Autodesk Inventor part; units mm, degrees
ref_plane "YZ Plane" through (0, 0, 0) normal (1, 0, 0) x (0, 1, 0)
ref_plane "XZ Plane" through (0, 0, 0) normal (0, 1, 0) x (-1, 0, 0)
ref_plane "XY Plane" through (0, 0, 0) normal (0, 0, 1) x (1, 0, 0)
sketch "Sketch1" plane through (0, 0, 0) normal (0, 1, 0) x (-1, 0, 0)
  line L0 (0, 0) -> (8, 0)
  line L1 (8, -30) -> (0, -30)
  line L2 (0, -30) -> (0, 0)
  line L3 (6.25, -3.4) -> (1.75, -3.4)
  line L4 (1.75, -3.4) -> (1.75, -6.4)
  line L5 (1.75, -6.4) -> (6.25, -6.4)
  line L6 (6.25, -6.4) -> (6.25, -3.4)
  line L7 (6.25, -23.6) -> (1.75, -23.6)
  line L8 (1.75, -23.6) -> (1.75, -26.6)
  line L9 (1.75, -26.6) -> (6.25, -26.6)
  line L10 (6.25, -26.6) -> (6.25, -23.6)
  line L11 (8, 0) -> (30, -7.5)
  line L12 (30, -7.5) -> (30, -22.5)
  line L13 (30, -22.5) -> (8, -30)
  dimension "d0" = 30
  dimension "d1" = 8
  dimension "d2" = 4.5
  dimension "d3" = 3
  dimension "d4" = 3
  dimension "d5" = 17.2
  dimension "d6" = 3.4
  dimension "d7" = 1.75
  dimension "d8" = 15
  dimension "d10" = 7.5
  dimension "d11" = 22
  dimension "d12" = 22
extrude "Extrusion1" add sketch "Sketch1" along normal blind 3
sketch "Sketch2" plane through (0, 3, 0) normal (0, 1, 0) x (1, 0, 0)
  circle A0 centre (-7, 15) radius 1.3
  line L0 (-30, 22.5) -> (-30, 7.5)
  line L1 (-30, 7.5) -> (0, 7.5)
  line L2 (-30, 22.5) -> (0, 22.5)
  line L3 (-30, 7.5) -> (-14.7467, 2.3)
  line L4 (-30, 7.5) -> (-8, 0)
  line L5 (0, 0) -> (0, 30)
  line L6 (0, 2.3) -> (0, 7.5)
  line L7 (0, 2.3) -> (-14.7467, 2.3)
  line L8 (-8, 30) -> (-30, 22.5)
  line L9 (-30, 22.5) -> (-14.7467, 27.7)
  line L10 (-14.7467, 27.7) -> (0, 27.7)
  line L11 (0, 27.7) -> (0, 22.5)
  line L12 (-8, 0) -> (0, 0)
  line L13 (-1.75, 3.4) -> (-6.25, 3.4)
  line L14 (-6.25, 26.6) -> (-1.75, 26.6)
  point P0 (0, 27.7)
  dimension "d17" = 2.6
  dimension "d21" = 1.1
  dimension "d22" = 1.1
  dimension "d23" = 15
  dimension "d24" = 7
extrude "Extrusion2" add sketch "Sketch2" along normal blind 7 contours A0 | L8 L10 L5 L2 | L1 L5 L7 L3
sketch "Sketch3" plane through (0, 0, 0) normal (0, -1, 0) x (1, 0, 0)
  line L0 (-1.75, -6.4) -> (-1.75, -3.4)
  line L1 (-1.75, -3.4) -> (-6.25, -3.4)
  line L2 (-6.25, -3.4) -> (-6.25, -6.4)
  line L3 (-6.25, -6.4) -> (-1.75, -6.4)
  line L4 (-1.75, -6.4) -> (-1.75, -3.4)
  line L5 (-1.75, -26.6) -> (-1.75, -23.6)
  line L6 (-6.25, -26.6) -> (-1.75, -26.6)
  line L7 (-1.75, -23.6) -> (-6.25, -23.6)
  line L8 (-6.25, -23.6) -> (-6.25, -26.6)
  line L9 (-6.25, -26.6) -> (-1.75, -26.6)
  line L10 (-1.75, -26.6) -> (-1.75, -23.6)
  point P0 (0, 0)
extrude "Extrusion3" cut sketch "Sketch3" against normal through all
sketch "Sketch4" plane through (0, 3, 0) normal (0, 1, 0) x (1, 0, 0)
  line L0 (0, 7.5) -> (0, 22.5)
  line L1 (0, 11) -> (-4, 11)
  line L2 (-4, 11) -> (-4, 19)
  line L3 (-4, 19) -> (0, 19)
  line L4 (0, 19) -> (0, 11)
  circle A0 centre (-7, 15) radius 1.3
  line L5 (0, 7.5) -> (-30, 7.5)
  point P0 (0, 0)
  point P1 (0, 19)
  dimension "d29" = 3
  dimension "d30" = 8
  dimension "d31" = 3.5
extrude "Extrusion4" cut sketch "Sketch4" against normal through all contours L1 L2 L3 L0
fillet "Fillet1" radius 1 1 edges at (-8.3, 3, -15)
properties part number "IRMount"
Could you check a few things on this model? Use its own coordinates, in mm. A direction names the side the tool comes from. Give positions to 0.01 mm unless a question says otherwise; leave off trailing zeros. Loops run counter-clockwise (first coordinate to the right, second up) from the corner with the lowest first, then second, coordinate; pieces in that order, holes last. Notation, with made-up numbers: (36.25, 2.5) - (92.25, 2.5) arc R18 ccw to (92.25, 19.5) - close; hole circle Ø7 at (80, -13). An arc over 180 degrees is marked (long way). Answer in a Markdown table with one row per item. Add a question column.
Q1. If we section it at D-D (y = 2.5): List the corners of the cut face in (x, z) for me.
Q2. For pin 1 (0.7 mm diameter, centred on x = -4, z = -1, fed in from +Y); pin 2 (2.5 mm diameter, centred on y = 2, z = -13, fed in from +X); pin 3 (1.3 mm diameter, centred on x = -4, y = 6, fed in from +Z); pin 4 (2 mm diameter, centred on y = 2.5, z = -21, fed in from +X), each with a flat end and sliding along its axis, tell me the tip position at first contact or that it passes through.
Q3. If we section it at C-C (x = -7): List the corners of the cut face in (y, z) for me.
Q4. If we section it at A-A (y = 4.75): List the corners of the cut face in (x, z) for me.
Q5. If we section it at B-B (z = -24): List the corners of the cut face in (x, y) for me.
Q6. Please list where these lines run through material, in increasing order: L1, parallel to Z at x = -2.5, y = 5.5; L2, parallel to Z at x = -8.5, y = 9.25; L3, parallel to Z at x = -6.75, y = 6.75. Write a range as from..to.
Q7. We'd pull the mould along Z, two halves only. Please class faces 4 (the face through (-6.25, 5, -25)), 5 (the face through (-4, 1, -30)), 6 (the face through (-15, 0, -15)): +Z half, -Z half, draft (parallel to the pull), parting line (faces both ways), or undercut.
Q8. Which directions (+Z, -Z, +X, -X, +Y, -Y) give clear straight access to the entire face, cutting with the end or side of a thin tool? Please do faces 1 (the face through (-15, 6, -7.5)), 2 (the face through (-1.75, 5, -5)), 3 (the face through (-6, 3, -29)).
The answers:
| question | item | result |
|---|---|---|
| 1 | outline | (-30, -22.5) - (-8, -30) - (0, -30) - (0, -19) - (-4, -19) - (-4, -11) - (0, -11) - (0, 0) - (-8, 0) - (-30, -7.5) - close; hole (-6.25, -26.6) - (-1.75, -26.6) - (-1.75, -23.6) - (-6.25, -23.6) - close; hole (-6.25, -6.4) - (-1.75, -6.4) - (-1.75, -3.4) - (-6.25, -3.4) - close |
| 2 | pin 1 | stops at y = 3 |
| 2 | pin 2 | stops at x = -4 |
| 2 | pin 3 | stops at z = -2.3 |
| 2 | pin 4 | stops at x = 0 |
| 3 | outline | (0, -30) - (3, -30) - (3, -27.7) - (10, -27.7) - (10, -22.5) - (3, -22.5) - (3, -17.3) arc R1 cw to (4, -16.3) - (10, -16.3) - (10, -13.7) - (4, -13.7) arc R1 cw to (3, -12.7) - (3, -7.5) - (10, -7.5) - (10, -2.3) - (3, -2.3) - (3, 0) - (0, 0) - close |
| 4 | outline | (-30, -22.5) - (-14.75, -27.7) - (0, -27.7) - (0, -22.5) - close; (-30, -7.5) - (0, -7.5) - (0, -2.3) - (-14.75, -2.3) - close; circle Ø2.6 at (-7, -15); hole (-6.25, -26.6) - (-1.75, -26.6) - (-1.75, -23.6) - (-6.25, -23.6) - close; hole (-6.25, -6.4) - (-1.75, -6.4) - (-1.75, -3.4) - (-6.25, -3.4) - close |
| 5 | outline | (-25.6, 0) - (-6.25, 0) - (-6.25, 10) - (-25.6, 10) - close; (-1.75, 0) - (0, 0) - (0, 10) - (-1.75, 10) - close |
| 6 | L1 | z = -27.7..-26.6, -23.6..-22.5, -7.5..-6.4, -3.4..-2.3 |
| 6 | L2 | z = -27.7..-22.5, -7.5..-2.3 |
| 6 | L3 | z = -27.7..-22.5, -16.28..-13.72, -7.5..-2.3 |
| 7 | face 4 | undercut |
| 7 | face 5 | -Z half |
| 7 | face 6 | draft |
| 8 | face 1 | +X, -X, +Y |
| 8 | face 2 | +Y, -Y |
| 8 | face 3 | -Z, +X, -X, +Y |
